```python
from build123d import *

# Parameters (mm, degrees)
SKETCH1_R           = 25.4
BOSS_EXTRUDE1_DEPTH = 76.2
SKETCH2_R           = 22.225
CUT_EXTRUDE1_DEPTH  = 69.85
CHAMFER1_SIZE       = 3.175
SKETCH3_R           = 1.5875
CUT_EXTRUDE2_DEPTH  = 63.5
SKETCH6_R           = 3.175
CUT_EXTRUDE3_DEPTH  = 51.8


with BuildPart() as part:
    # Sketch1 → Boss-Extrude1 (new body)
    with BuildSketch(Plane(origin=(0, 0, 0), x_dir=(1, 0, 0), z_dir=(0, 1, 0))):
        Circle(SKETCH1_R)
    extrude(amount=BOSS_EXTRUDE1_DEPTH)

    # Sketch2 → Cut-Extrude1 (cut)
    with BuildSketch(Plane(origin=(0, 76.2, 0), x_dir=(1, 0, 0), z_dir=(0, 1, 0))):
        Circle(SKETCH2_R)
    extrude(amount=-CUT_EXTRUDE1_DEPTH, mode=Mode.SUBTRACT)

    # Chamfer1
    chamfer1_edges = [part.edges().sort_by_distance(p)[0] for p in [
        (-25.4, 0, 0),
    ]]
    chamfer(chamfer1_edges, length=CHAMFER1_SIZE)

    # Sketch3 → Cut-Extrude2 (cut)
    with BuildSketch(Plane(origin=(0, 6.35, 0), x_dir=(1, 0, 0), z_dir=(0, 1, 0))):
        with Locations((-12.7, 0)):
            Circle(SKETCH3_R)
        with Locations((12.7, 0)):
            Circle(SKETCH3_R)
    extrude(amount=-CUT_EXTRUDE2_DEPTH, mode=Mode.SUBTRACT)

    # Sketch6 → Cut-Extrude3 (cut, through all)
    with BuildSketch(Plane.XY.offset(25.4)):
        with Locations((0, 23.8125)):
            Circle(SKETCH6_R)
        with Locations((0, 58.7375)):
            Circle(SKETCH6_R)
    extrude(amount=-CUT_EXTRUDE3_DEPTH, mode=Mode.SUBTRACT)


solid = part.part
```
Here's how the part is built. I have some questions about the finished solid (model axes, mm). A direction names the side the tool comes from. Round coordinates to 2 decimals unless told otherwise and drop trailing zeros. Write each loop counter-clockwise with the first axis right and the second up, starting at its lowest first coordinate (ties: lowest second). Pieces come first, ordered by that corner, then holes.
Q1. If we section it at D-D on y = 46: Write out the boundary of the cut face in (x, z) (3 decimals).
Q2. Please list where these lines run through material, in increasing order: probe 1 along X at (y, z) = (4, 0); probe 2 along Y at (x, z) = (0, -24) (1 decimal); probe 3 along Y at (x, z) = (0, 23) (1 decimal).
Q3. If we section it at A-A on x = 0: Give the number of separate pieces and of enclosed holes in the cut face, plus the area to 3 significant figures.
Q4. If we section it at C-C on y = 57: Write out the boundary of the cut face in (x, z) (3 decimals), plus the area to 3 significant figures.
Q5. If we mould it in two halves opening along Z, with no side actions, what happens to faces 3 (the flat face through (-0.1, 76.2, 22.5)), 4 (the cylindrical face through (-11.186, 3.219, -0.477)), 5 (the cylindrical face through (-5.506, 39.176, 24.796))? For each: +Z half, -Z half, draft (parallel to the pull), parting line (faces both ways), or undercut.
Q6. Will these pins go through, and if not, where does the flat tip stop? P1, Ø12, axis at x = 4.5, z = 3.5, coming from the +Y side; P2, Ø5, axis at y = 44.5, z = -13, coming from the -X side; P3, Ø1, axis at y = 13.5, z = 2, coming from the -X side; P4, Ø3, axis at x = -12.7, z = 0, coming from the -Y side.
Q7. Which directions (+Z, -Z, +X, -X, +Y, -Y) give clear straight access to the entire face, cutting with the end or side of a thin tool? Please do faces 1 (the cylindrical face through (21.199, 41.764, -6.676)), 2 (the cylindrical face through (-0.413, 61.885, -23.676)).
Answer below:
1. outline: circle Ø50.8 at (0, 0); hole circle Ø44.45 at (0, 0)
2. probe 1: x = -25.4 to -14.29, -11.11 to 11.11, 14.29 to 25.4
2. probe 2: y = 1.8 to 20.6, 27 to 55.6, 61.9 to 76.2
2. probe 3: y = 0.8 to 20.6, 27 to 55.6, 61.9 to 76.2
3. separate pieces: 5
3. enclosed holes: 0
3. area: 675 mm2
4. outline: (-2.657, -25.261) - (-2.657, -22.066) arc R22.225 cw to (-2.657, 22.066) - (-2.657, 25.261) arc R25.4 ccw to start; (2.657, -25.261) arc R25.4 ccw to (2.657, 25.261) - (2.657, 22.066) arc R22.225 cw to (2.657, -22.066) - close
4. area: 441 mm2
5. face 3: draft
5. face 4: undercut
5. face 5: parting line
6. P1: stops at y = 6.35
6. P2: stops at x = -23.13
6. P3: stops at x = -25.36
6. P4: passes through
7. face 1: +Y
7. face 2: +Z, -Z
